Verification items for the finished model (mm, model axes). A direction names the side the tool comes from. Give positions to 0.01 mm unless a question says otherwise; leave off trailing zeros. Write each loop counter-clockwise with the first axis right and the second up, starting at its lowest first coordinate (ties: lowest second). Pieces come first, ordered by that corner, then holes. Notation, with made-up numbers: M 58,-39 L 69,-39 A25 ccw 69,-9 Z; hole C 75.5,7 d7. An arc over 180 degrees is marked long. Answer as a JSON object with one key per item and string values.
```python
from build123d import *

# Parameters (mm, degrees)
SKETCH_1_W            = 17
SKETCH_1_H            = 18
EXTRUDE_1_DEPTH       = 1
SKETCH_2_R            = 1
CUT_EXTRUDE_1_DEPTH   = 13.419742348
CUT_EXTRUDE_2_DEPTH   = 13.419742348
MIRROR_2_COPY_1_DEPTH = 13.419742348
SKETCH_4_W            = 5
SKETCH_4_H            = 3
CUT_EXTRUDE_3_DEPTH   = 13.419742348
EXTRUDE_2_DEPTH       = 1
EXTRUDE_3_DEPTH       = 1
EXTRUDE_START         = 8.5
SKETCH_8_W            = 8.3
SKETCH_8_H            = 3.1
EXTRUDE_4_DEPTH       = 4.2
SKETCH_9_W            = 10.2
SKETCH_9_H            = 9
EXTRUDE_5_DEPTH       = 2
SKETCH_10_R           = 1.5
EXTRUDE_10_DEPTH      = 100


with BuildPart() as part:
    # 草图1 → 凸台-拉伸1 (new body)
    with BuildSketch(Plane(origin=(0, 0, 0), x_dir=(1, 0, 0), z_dir=(0, 1, 0))):
        Rectangle(SKETCH_1_W, SKETCH_1_H)
    extrude(amount=EXTRUDE_1_DEPTH)

    # 草图2 → 切除-拉伸1 (cut, through all)
    with BuildSketch(Plane(origin=(0, 1, 0), x_dir=(1, 0, 0), z_dir=(0, 1, 0))):
        with Locations(Location((-5.5, 7, 0), (0, 0, 270))):
            Circle(SKETCH_2_R)
        with Locations(Location((5.5, 7, 0), (0, 0, 270))):
            Circle(SKETCH_2_R)
        with Locations(Location((-5.5, -7, 0), (0, 0, 270))):
            Circle(SKETCH_2_R)
        with Locations(Location((5.5, -7, 0), (0, 0, 270))):
            Circle(SKETCH_2_R)
    extrude(amount=-CUT_EXTRUDE_1_DEPTH, mode=Mode.SUBTRACT)

    # 草图3 → 切除-拉伸2 (cut, through all)
    with BuildSketch(Plane(origin=(0, 1, 0), x_dir=(1, 0, 0), z_dir=(0, 1, 0))):
        with BuildLine():
            Line((-8.5, 9), (-8.5, 6))
            ThreePointArc((-8.5, 6), (-7.621320346, 8.121320341), (-5.500000007, 9))
            Line((-5.500000007, 9), (-8.5, 9))
        make_face()
        with BuildLine():
            Line((-2.5, 9), (-5.500000007, 9))
            ThreePointArc((-5.500000007, 9), (-3.378679659, 8.121320346), (-2.5, 6))
            Line((-2.5, 6), (-2.5, 9))
        make_face()
    cut_extrude_2 = extrude(amount=-CUT_EXTRUDE_2_DEPTH, mode=Mode.SUBTRACT)

    # 镜向1: 切除-拉伸2 across plane
    add(cut_extrude_2.mirror(Plane.XY), mode=Mode.SUBTRACT)

    # 镜向2: 切除-拉伸2 across plane
    add(cut_extrude_2.mirror(Plane(origin=(0, 0, 0), x_dir=(0, 0, 1), z_dir=(1, 0, 0))), mode=Mode.SUBTRACT)

    # 镜向2 copy 1 sketch → 镜向2 copy 1 (cut, through all)
    with BuildSketch(Plane(origin=(0, 1, 0), x_dir=(-1, 0, 0), z_dir=(0, 1, 0))):
        with BuildLine():
            Line((-8.5, 9), (-8.5, 6))
            ThreePointArc((-8.5, 6), (-7.621320346, 8.121320341), (-5.500000007, 9))
            Line((-5.500000007, 9), (-8.5, 9))
        make_face()
        with BuildLine():
            Line((-2.5, 9), (-5.500000007, 9))
            ThreePointArc((-5.500000007, 9), (-3.378679659, 8.121320346), (-2.5, 6))
            Line((-2.5, 6), (-2.5, 9))
        make_face()
    extrude(amount=-MIRROR_2_COPY_1_DEPTH, mode=Mode.SUBTRACT)

    # 草图4 → 切除-拉伸3 (cut, through all)
    with BuildSketch(Plane(origin=(0, 1, 0), x_dir=(1, 0, 0), z_dir=(0, 1, 0))):
        with Locations((0, 7.5)):
            Rectangle(SKETCH_4_W, SKETCH_4_H)
    cut_extrude_3 = extrude(amount=-CUT_EXTRUDE_3_DEPTH, mode=Mode.SUBTRACT)

    # 镜向3: 切除-拉伸3 across plane
    add(cut_extrude_3.mirror(Plane.XY), mode=Mode.SUBTRACT)

    # 草图5 → 凸台-拉伸2 (add)
    with BuildSketch(Plane(origin=(0, 1, 0), x_dir=(1, 0, 0), z_dir=(0, 1, 0))):
        with BuildLine():
            Line((0, 0), (-2.3, 3.5))
            ThreePointArc((-2.3, 3.5), (-5.8, 0), (-2.3, -3.5))
            Line((-2.3, -3.5), (0, 0))
        make_face()
        Polygon((2.3, 3.5), (-2.3, 3.5), (0, 0), align=None)
        Polygon((2.3, -3.5), (0, 0), (-2.3, -3.5), align=None)
        with BuildLine():
            ThreePointArc((2.3, -3.5), (5.8, 0), (2.3, 3.5))
            Line((2.3, 3.5), (0, 0))
            Line((0, 0), (2.3, -3.5))
        make_face()
    extrude(amount=EXTRUDE_2_DEPTH)

    # 草图6 → 凸台-拉伸3 (add)
    with BuildSketch(Plane(origin=(0, 2, 0), x_dir=(1, 0, 0), z_dir=(0, 1, 0))):
        with BuildLine():
            Line((0, 0), (-2.3, 2.5))
            ThreePointArc((-2.3, 2.5), (-4.8, 0), (-2.3, -2.5))
            Line((-2.3, -2.5), (0, 0))
        make_face()
        Polygon((2.3, 2.5), (-2.3, 2.5), (0, 0), align=None)
        Polygon((2.3, -2.5), (0, 0), (-2.3, -2.5), align=None)
        with BuildLine():
            ThreePointArc((2.3, -2.5), (4.8, 0), (2.3, 2.5))
            Line((2.3, 2.5), (0, 0))
            Line((0, 0), (2.3, -2.5))
        make_face()
    extrude(amount=EXTRUDE_3_DEPTH)

    # 草图8 → 凸台-拉伸4 (add)
    with BuildSketch(Plane(origin=(0, 0, 0), x_dir=(0, 0, -1), z_dir=(1, 0, 0)).offset(EXTRUDE_START)):
        with Locations((0, -1.55)):
            Rectangle(SKETCH_8_W, SKETCH_8_H)
    extrude(amount=-EXTRUDE_4_DEPTH)

    # 草图9 → 凸台-拉伸5 (add)
    with BuildSketch(Plane.XZ):
        with Locations((-2.21638326, 0)):
            Rectangle(SKETCH_9_W, SKETCH_9_H)
    extrude(amount=EXTRUDE_5_DEPTH)

    # 草图10 → 凸台-拉伸10 (add)
    with BuildSketch(Plane(origin=(0, 3, 0), x_dir=(1, 0, 0), z_dir=(0, 1, 0))):
        with Locations(Location((0, 0, 0), (0, 0, 270))):
            Circle(SKETCH_10_R)
    extrude(amount=EXTRUDE_10_DEPTH)


solid = part.part
```
1) Section check C-C on z = -7. Record the boundary of the cut face in (x, y).
Completed:
{"outline": "M -8.33,0 L -6.5,0 L -6.5,1 L -8.33,1 Z; M -4.5,0 L -2.67,0 L -2.67,1 L -4.5,1 Z; M 2.67,0 L 4.5,0 L 4.5,1 L 2.67,1 Z; M 6.5,0 L 8.33,0 L 8.33,1 L 6.5,1 Z"}
2) Section check B-B on x = 0. Record the boundary of the cut face in (y, z), and give its area (3 significant figures).
Completed:
{"outline": "M -2,-4.5 L 0,-4.5 L 0,-6 L 1,-6 L 1,-3.5 L 2,-3.5 L 2,-2.5 L 3,-2.5 L 3,-1.5 L 103,-1.5 L 103,1.5 L 3,1.5 L 3,2.5 L 2,2.5 L 2,3.5 L 1,3.5 L 1,6 L 0,6 L 0,4.5 L -2,4.5 Z", "area": "342 mm2"}
3) Thickness scan on L1, parallel to X at y = 0.3, z = 7; L2, parallel to Y at x = 3, z = -7; L3, parallel to Y at x = 7.5, z = 2.75. Record the ranges inside material, lowest first.
Completed:
{"L1": "x = -8.33 to -6.5, -4.5 to -2.67, 2.67 to 4.5, 6.5 to 8.33", "L2": "y = 0 to 1", "L3": "y = -3.1 to 1"}
4) Access from +Z, -Z, +X, -X, +Y, -Y to the whole of each face (thin tool, end or side, straight path). Record for faces 5 (the face through (-2, -1, -4.5)), 6 (the face through (0.45, 52.3, 1.43)), 7 (the face through (-2, -1, 4.5)), 8 (the face through (-5.8, 1.5, -0.1)).
Completed:
{"face 5": "-Z, +X, -X, -Y", "face 6": "+Y", "face 7": "+Z, +X, -X, -Y", "face 8": "-X, +Y"}
5) Section check A-A on z = 0. Record the boundary of the cut face in (x, y).
Completed:
{"outline": "M -8.5,0 L -7.32,0 L -7.32,-2 L 2.88,-2 L 2.88,0 L 4.3,0 L 4.3,-3.1 L 8.5,-3.1 L 8.5,1 L 5.8,1 L 5.8,2 L 4.8,2 L 4.8,3 L 1.5,3 L 1.5,103 L -1.5,103 L -1.5,3 L -4.8,3 L -4.8,2 L -5.8,2 L -5.8,1 L -8.5,1 Z"}
6) Release check for a two-part mould opening along X. For faces 1 (the face through (5.8, 1.5, 0.1)), 2 (the face through (4.3, -2, 0)), 3 (the face through (-4.8, 2.5, -0.1)), 4 (the face through (2.884, -1, 0)) record: pulls with the +X half, pulls with the -X half, needs draft (parallel to the pull), parting line crosses it, or undercut.
Completed:
{"face 1": "pulls with the +X half", "face 2": "undercut", "face 3": "pulls with the -X half", "face 4": "undercut"}
7) Go/stop test with flat-tipped pins: pin 1 (0.6 mm diameter, centred on x = -3, y = -1, fed in from -Z); pin 2 (5 mm diameter, centred on x = 3, z = -6.5, fed in from -Y); pin 3 (6 mm diameter, centred on x = -5.5, z = -4, fed in from +Y); pin 4 (3.5 mm diameter, centred on x = 6, y = -1, fed in from +Z). Record where each tip stops, or that it passes through.
Completed:
{"pin 1": "stops at z = -4.5", "pin 2": "stops at y = -2", "pin 3": "stops at y = 3", "pin 4": "stops at z = 9"}
8) Section check D-D on y = 33. Record the boundary of the cut face in (x, z), and give its area (3 significant figures).
Completed:
{"outline": "C 0,0 d3", "area": "7.07 mm2"}
